Could you check a few things on this model? Use its own coordinates, in mm. A direction names the side the tool comes from. Coordinates: 2 decimals unless noted, no trailing zeros. Loops run counter-clockwise (first coordinate to the right, second up) from the corner with the lowest first, then second, coordinate; pieces in that order, holes last. Notation, with made-up numbers: (79.25, 44.25) - (104.25, 44.25) arc R19 ccw to (104.25, 49.25) - close; hole circle Ø6 at (29, -4). An arc over 180 degrees is marked (long way). One line per item, written item: value. Start each with the question number.
(1) If we mould it in two halves opening along Y, with no side actions, what happens to faces 4 (the face through (47, 0, 150)), 5 (the face through (47, 95.25, 150)), 6 (the face through (14, 28.575, 257)), 7 (the face through (28.575, 14, 257))? For each: pulls with the +Y half, pulls with the -Y half, needs draft (parallel to the pull), parting line crosses it, or undercut.
(2) If we section it at A-A on z = 231: Write out the boundary of the cut face in (x, y) (3 decimals).
(3) If we section it at B-B on x = 18.5: Write out the boundary of the cut face in (y, z) (3 decimals).
(4) I'm going to push flat-ended pins straight in: P1, Ø8.5, axis at y = 86.5, z = 270, coming from the -X side; P2, Ø5, axis at x = 33, y = 30, coming from the +Z side. Where does each tip first touch, or does it pass through?
(5) On a 3-axis mill with a long thin cutter (end or side, diameter ignored), from which of +Z, -Z, +X, -X, +Y, -Y can I reach the whole of each face in a straight line? I mean faces 1 (the face through (14, 66.675, 257)), 2 (the face through (47, 48, 0)), 3 (the face through (66.675, 81, 257)). Say none if no direction works.
(6) If we section it at D-D on y = 59: Write out the boundary of the cut face in (x, z).
(7) If I drill on line 1 along Y through (x, z) = (71, 292) (3 decimals); line 2 along Z through (x, y) = (59.5, 38.5), over which ranges is the centre line in solid material (lowest first)? Write a range as from..to.
```python
from build123d import *

# Parameters (mm, degrees)
F0_W     = 95.25
F0_H     = 95.25
F2_DEPTH = 304.8
F3_START = 209.55
F1_W     = 28.575
F1_H     = 38.1
F1_W_2   = 38.1
F1_H_2   = 28.575
F3_DEPTH = 95.25


with BuildPart() as f2:
    # F0 (on Top) → F2 (new body)
    with BuildSketch(Plane.XY):
        with Locations((47.625, 47.625)):
            Rectangle(F0_W, F0_H)
    extrude(amount=F2_DEPTH)

    # F1 (on Top) → F3 (cut)
    with BuildSketch(Plane.XY.offset(F3_START)):
        with Locations((14.2875, 47.625)):
            Rectangle(F1_W, F1_H)
        with Locations((47.625, 47.625)):
            Rectangle(F1_W_2, F1_H)
        with Locations((80.9625, 47.625)):
            Rectangle(F1_W, F1_H)
        with Locations((47.625, 80.9625)):
            Rectangle(F1_W_2, F1_H_2)
        with Locations((47.625, 14.2875)):
            Rectangle(F1_W_2, F1_H_2)
    extrude(amount=F3_DEPTH, mode=Mode.SUBTRACT)


solid = f2.part
```
Values:
1. face 4: pulls with the -Y half
1. face 5: pulls with the +Y half
1. face 6: undercut
1. face 7: needs draft
2. outline: (0, 0) - (28.575, 0) - (28.575, 28.575) - (0, 28.575) - close; (0, 66.675) - (28.575, 66.675) - (28.575, 95.25) - (0, 95.25) - close; (66.675, 0) - (95.25, 0) - (95.25, 28.575) - (66.675, 28.575) - close; (66.675, 66.675) - (95.25, 66.675) - (95.25, 95.25) - (66.675, 95.25) - close
3. outline: (0, 0) - (95.25, 0) - (95.25, 304.8) - (66.675, 304.8) - (66.675, 209.55) - (28.575, 209.55) - (28.575, 304.8) - (0, 304.8) - close
4. P1: stops at x = 0
4. P2: stops at z = 209.55
5. face 1: +Z, +X, -X
5. face 2: -Z, +X, -X, +Y, -Y
5. face 3: +Z, +Y, -Y
6. outline: (0, 0) - (95.25, 0) - (95.25, 209.55) - (0, 209.55) - close
7. line 1: y = 0..28.575, 66.675..95.25
7. line 2: z = 0..209.55
